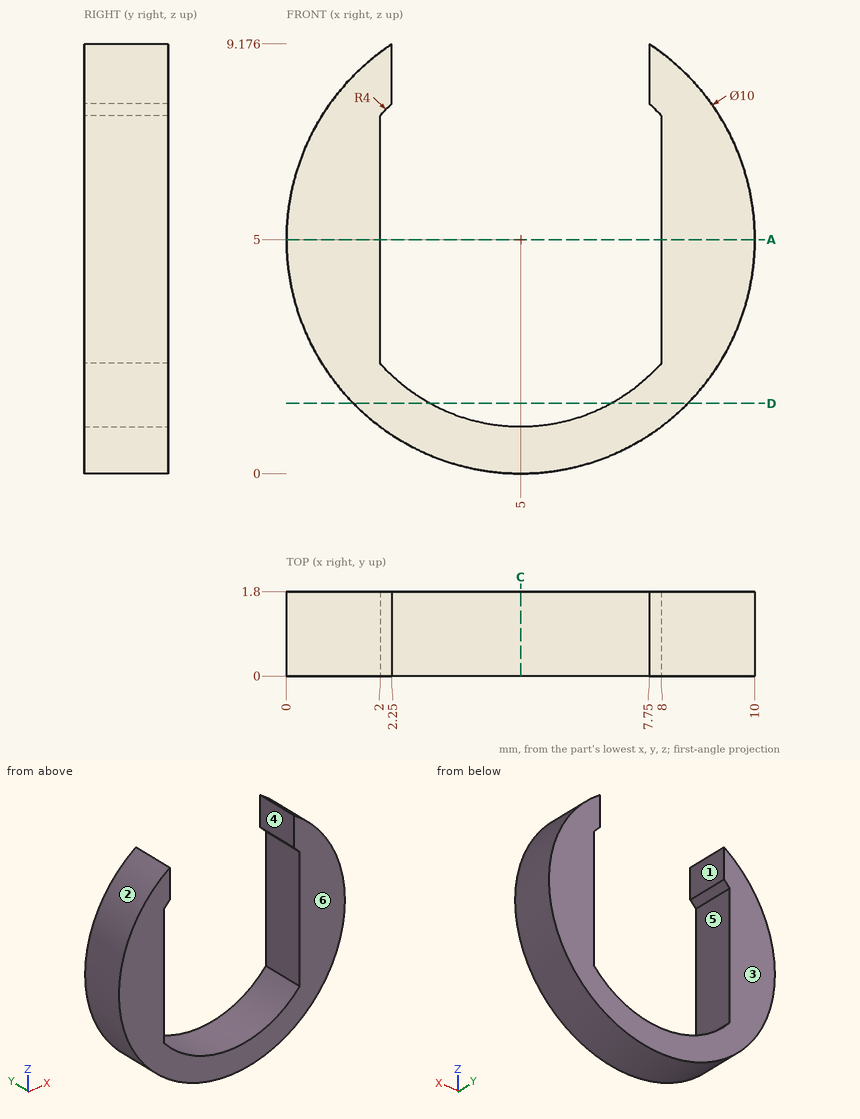
For this review, use the dimensioned drawing (mm, ordinates from the lowest corner) and the shaded views. A direction names the side the tool comes from. Coordinates: 2 decimals unless noted, no trailing zeros. Loops run counter-clockwise (first coordinate to the right, second up) from the corner with the lowest first, then second, coordinate; pieces in that order, holes last. Notation, with made-up numbers: (-28, 43) -> (2, 43) arc R29 cw to (2, 68) -> close; hole circle Ø3 at (37.25, 9). An arc over 180 degrees is marked (long way). Use a Markdown table: item, result. Add a question column.
1. Draft analysis for pull direction X (two halves, no side actions). For the marked faces 1, 2 and 3, state which applies: pulls with the +X half, pulls with the -X half, needs draft (parallel to the pull), parting line crosses it, or undercut.
2. Add section A-A on z = 5. Write out the cut boundary in (x, y).
3. Machinability: for the marked faces 4, 5 and 6, which of the approach directions +Z, -Z, +X, -X, +Y, -Y give a long, thin tool a straight path to every point of the face, cutting with its end or side? Answer none if there is none.
4. Add section C-C on x = 5. Write out the cut boundary in (y, z).
5. Add section D-D on z = 1.5. Write out the cut boundary in (x, y).
6. To check wall thickness, follow line 1 (X direction, y = 0.3, z = 8.5); line 2 (X direction, y = 0.2, z = 7.5); line 3 (Z direction, x = 5, y = 0.55). State the ranges of each line that lie inside material, in increasing order.
7. Clearance check with flat-ended pins moving along their axes: pin 1 Ø0.6 at (y, z) = (1.5, 8.5) entering from +X; pin 2 Ø0.6 at (y, z) = (1, 8.5) entering from -X; pin 3 Ø1 at (y, z) = (0.5, 8) entering from -X. State where each tip first meets the part, or that it passes through.
Returned:
| question | item | result |
|---|---|---|
| 1 | face 1 | undercut |
| 1 | face 2 | parting line crosses it |
| 1 | face 3 | needs draft |
| 2 | outline | (0, 0) -> (2, 0) -> (2, 1.8) -> (0, 1.8) -> close; (8, 0) -> (10, 0) -> (10, 1.8) -> (8, 1.8) -> close |
| 3 | face 4 | +Z, +Y, -Y |
| 3 | face 5 | +Y, -Y |
| 3 | face 6 | +Z, -Z, +X, -X, -Y |
| 4 | outline | (0, 0) -> (1.8, 0) -> (1.8, 1) -> (0, 1) -> close |
| 5 | outline | (1.43, 0) -> (3.06, 0) -> (3.06, 1.8) -> (1.43, 1.8) -> close; (6.94, 0) -> (8.57, 0) -> (8.57, 1.8) -> (6.94, 1.8) -> close |
| 6 | line 1 | x = 1.43 to 2.25, 7.75 to 8.57 |
| 6 | line 2 | x = 0.67 to 2, 8 to 9.33 |
| 6 | line 3 | z = 0 to 1 |
| 7 | pin 1 | stops at x = 8.84 |
| 7 | pin 2 | stops at x = 1.16 |
| 7 | pin 3 | stops at x = 0.67 |
